CAD build for the part. Positions are in the model's coordinates, mm. Round coordinates to 2 decimals unless told otherwise and drop trailing zeros. Write each loop counter-clockwise with the first axis right and the second up, starting at its lowest first coordinate (ties: lowest second). Pieces come first, ordered by that corner, then holes. Notation, with made-up numbers: (83.25, 55) - (113.25, 55) arc R22 ccw to (113.25, 70) - close; hole circle Ø10 at (68, 1.25). An arc over 180 degrees is marked (long way). Put each result on its own line as item: value. Start each with the question number.
Item 1: Cut at B-B (z = -8). Give the cut face in (x, y).
Item 2: Cut at D-D (z = -2). Give the cut face in (x, y).
Item 3: Cut at A-A (y = 12.75). Count the separate pieces of the cut face and the enclosed holes in it, and give its area (3 significant figures).
Item 4: Drill centre lines: line 1 (Y direction, x = 47, z = -16.5); line 2 (X direction, y = 3.75, z = -4.75); line 3 (X direction, y = 11.25, z = -28). Where is each one in solid material? Low to high. Write a range as from..to.
Item 5: Cut at C-C (x = 51). Give the cut face in (y, z).
Item 6: Pin check, flat tips, straight feed: pin 1 Ø8 at (x, y) = (50.5, 12.5) entering from -Z; pin 2 Ø0.6 at (y, z) = (12, -26) entering from -X; pin 3 Ø9 at (x, z) = (34, -20) entering from +Y; pin 4 Ø0.5 at (x, z) = (57.5, -26) entering from +Y. Stop position of each tip, or through.
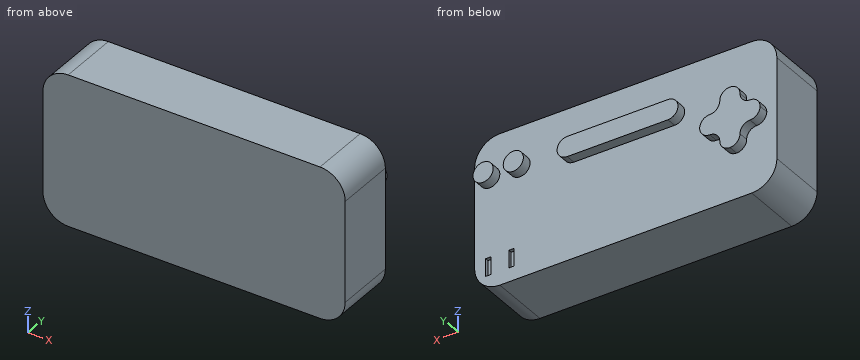
```python
from build123d import *

# Parameters (mm, degrees)
BOSS_EXTRUDE1_DEPTH = 12
SKETCH2_R           = 2
BOSS_EXTRUDE2_DEPTH = 2
SKETCH3_W           = 1
SKETCH3_H           = 3.5
CUT_EXTRUDE1_DEPTH  = 0.7
FILLET2_R           = 2


with BuildPart() as part:
    # Sketch1 → Boss-Extrude1 (new body)
    with BuildSketch(Plane(origin=(0, 0, 0), x_dir=(1, 0, 0), z_dir=(0, 1, 0))):
        with BuildLine():
            Line((5, 0), (55, 0))
            ThreePointArc((55, 0), (58.535533906, 1.464466094), (60, 5))
            Line((60, 5), (60, 25))
            ThreePointArc((60, 25), (58.535533906, 28.535533906), (55, 30))
            Line((55, 30), (5, 30))
            ThreePointArc((5, 30), (1.464466094, 28.535533906), (0, 25))
            Line((0, 25), (0, 5))
            ThreePointArc((0, 5), (1.464466094, 1.464466094), (5, 0))
        make_face()
    extrude(amount=BOSS_EXTRUDE1_DEPTH)

    # Sketch2 → Boss-Extrude2 (add)
    with BuildSketch(Plane(origin=(0, 12, 0), x_dir=(1, 0, 0), z_dir=(0, 1, 0))):
        with Locations(Location((57, 8, 0), (0, 0, 90))):
            Circle(SKETCH2_R)
        with Locations(Location((51, 8, 0), (0, 0, 90))):
            Circle(SKETCH2_R)
        Polygon((2, 17), (2, 13), (6, 13), (6, 9), (10, 9), (10, 13), (14, 13), (14, 17), (10, 17), (10, 21), (6, 21), (6, 17), align=None)
        with BuildLine():
            Line((20.303338261, 11), (40.303338261, 11))
            ThreePointArc((40.303338261, 11), (42.303338261, 9), (40.303338261, 7))
            Line((40.303338261, 7), (20.303338261, 7))
            ThreePointArc((20.303338261, 7), (18.303338261, 9), (20.303338261, 11))
        make_face()
    extrude(amount=BOSS_EXTRUDE2_DEPTH)

    # Sketch3 → Cut-Extrude1 (cut)
    with BuildSketch(Plane(origin=(0, 12, 0), x_dir=(1, 0, 0), z_dir=(0, 1, 0))):
        with Locations((52.7, 25.5)):
            Rectangle(SKETCH3_W, SKETCH3_H)
        with Locations((57.3, 25.5)):
            Rectangle(SKETCH3_W, SKETCH3_H)
    extrude(amount=-CUT_EXTRUDE1_DEPTH, mode=Mode.SUBTRACT)

    # Fillet2
    fillet2_edges = [part.edges().sort_by_distance(p)[0] for p in [
        (6, 13, -9),
        (6, 13, -13),
        (2, 13, -13),
        (2, 13, -17),
        (6, 13, -17),
        (6, 13, -21),
        (10, 13, -21),
        (10, 13, -17),
        (14, 13, -17),
        (14, 13, -13),
        (10, 13, -13),
        (10, 13, -9),
    ]]
    fillet(fillet2_edges, radius=FILLET2_R - 0.0001)  # a hair under: the kernel refuses the full size


solid = part.part
```
Output values:
1. outline: (0, 0) - (60, 0) - (60, 12) - (59, 12) - (59, 14) - (55, 14) - (55, 12) - (53, 12) - (53, 14) - (49, 14) - (49, 12) - (42.04, 12) - (42.04, 14) - (18.57, 14) - (18.57, 12) - (0, 12) - close
2. outline: (1, 0) - (59, 0) - (59, 12) - (1, 12) - close
3. separate pieces: 4
3. enclosed holes: 0
3. area: 194 mm2
4. line 1: 0..12
4. line 2: 0.01..59.99
4. line 3: 1..59
5. outline: (0, -30) - (12, -30) - (12, -10) - (14, -10) - (14, -6) - (12, -6) - (12, 0) - (0, 0) - close
6. pin 1: z = -30
6. pin 2: x = 0.05
6. pin 3: y = 12
6. pin 4: y = 11.3
